For this review, take the finished solid that the model builds, in its own axes (mm). Face numbers are marked on the shaded views. A direction names the side the tool comes from. Round coordinates to 2 decimals unless told otherwise and drop trailing zeros. Loops run counter-clockwise (first coordinate to the right, second up) from the corner with the lowest first, then second, coordinate; pieces in that order, holes last. Notation, with made-up numbers: M 23.5,61 L 44.5,61 A12 ccw 44.5,82 Z; hole C 8.25,-26 d4. An arc over 180 degrees is marked long. Write item = value, one per line. Start each with the question number.
Autodesk Inventor part; units mm, degrees
ref_plane "YZ Plane" through (0, 0, 0) normal (1, 0, 0) x (0, 1, 0)
ref_plane "XZ Plane" through (0, 0, 0) normal (0, 1, 0) x (-1, 0, 0)
ref_plane "XY Plane" through (0, 0, 0) normal (0, 0, 1) x (1, 0, 0)
sketch "Sketch1" plane through (0, 0, 0) normal (0, 0, 1) x (1, 0, 0)
  line L0 (-11.1369, 11.1369) -> (11.1369, 11.1369) construction
  line L1 (11.1369, 11.1369) -> (11.1369, -11.1369) construction
  line L2 (11.1369, -11.1369) -> (-11.1369, -11.1369) construction
  line L3 (-11.1369, -11.1369) -> (-11.1369, 11.1369) construction
  line L4 (-11.1369, 11.1369) -> (11.1369, -11.1369) construction
  line L5 (11.1369, 11.1369) -> (-11.1369, -11.1369) construction
  circle A0 centre (-11.1369, 11.1369) radius 3
  circle A1 centre (11.1369, 11.1369) radius 3
  circle A2 centre (-11.1369, -11.1369) radius 3
  circle A3 centre (0, -15.6056) radius 3
  circle A4 centre (11.1369, -11.1369) radius 3
  line L6 (-11.1369, -11.1369) -> (0, -15.6056) construction
  line L7 (0, -15.6056) -> (11.1369, -11.1369) construction
  line L8 (0, 0) -> (0, 30.7503) construction
  circle A5 centre (-11.1369, 11.1369) radius 6
  circle A6 centre (-11.1369, -11.1369) radius 6
  circle A7 centre (11.1369, -11.1369) radius 6
  circle A8 centre (11.1369, 11.1369) radius 6
  line L9 (-19.2384, -29.2384) -> (19.2384, -29.2384)
  line L10 (29.2384, -19.2384) -> (29.2384, 19.2384)
  line L11 (19.2384, 29.2384) -> (-19.2384, 29.2384)
  line L12 (-29.2384, 19.2384) -> (-29.2384, -19.2384)
  line L13 (-29.2384, -29.2384) -> (29.2384, 29.2384) construction
  line L14 (29.2384, -29.2384) -> (-29.2384, 29.2384) construction
  line L15 (-29.2384, 19.2384) -> (-19.2384, 29.2384)
  line L16 (19.2384, 29.2384) -> (29.2384, 19.2384)
  line L17 (29.2384, -19.2384) -> (19.2384, -29.2384)
  line L18 (-19.2384, -29.2384) -> (-29.2384, -19.2384)
  circle A9 centre (0, 0) radius 35 construction
  point P0 (0, 0)
  point P1 (25, 0)
  point P2 (0, 0)
  dimension "d31" = 70
  dimension "d2" = 31.5
  dimension "d4" = 6
  dimension "d5" = 6
  dimension "d6" = 12
  dimension "d18" = 12
  dimension "d21" = 10
  dimension "d22" = 10
  dimension "d23" = 10
  dimension "d24" = 10
  dimension "d25" = 10
  dimension "d26" = 10
  dimension "d27" = 10
  dimension "d28" = 10
extrude "Extrusion1" add sketch "Sketch1" against normal blind 10 contours A5 | A6 | A7 | A8 | L18 L12 L15 L11 L16 L10 L17 L9
extrude "Extrusion3" cut sketch "Sketch1" against normal blind 5 contours A0 | A1 | A2 | A4 | A5 | A6 | A7 | A8
sketch "Sketch3" plane through (0, 0, 0) normal (0, 0, 1) x (1, 0, 0)
  circle A0 centre (-11.1369, -11.1369) radius 6
  circle A1 centre (11.1369, -11.1369) radius 6
  circle A2 centre (-11.1369, 11.1369) radius 6
  circle A3 centre (11.1369, 11.1369) radius 6
  line L0 (-29.2384, -19.2384) -> (-19.2384, -29.2384)
  line L1 (-19.2384, -29.2384) -> (19.2384, -29.2384)
  line L2 (19.2384, -29.2384) -> (29.2384, -19.2384)
  line L3 (29.2384, -19.2384) -> (29.2384, 19.2384)
  line L4 (29.2384, 19.2384) -> (19.2384, 29.2384)
  line L5 (19.2384, 29.2384) -> (-19.2384, 29.2384)
  line L6 (-19.2384, 29.2384) -> (-29.2384, 19.2384)
  line L7 (-29.2384, 19.2384) -> (-29.2384, -19.2384)
  circle A4 centre (0, -15.6056) radius 3
  line L8 (19.2384, 29.2384) -> (16.41, 26.41)
  line L9 (13.5815, 23.5815) -> (23.5815, 13.5815)
  line L10 (23.5815, 13.5815) -> (26.41, 16.41) construction
  line L11 (29.2384, 19.2384) -> (29.2384, -19.2384)
  line L12 (29.2384, 19.2384) -> (19.2384, 29.2384)
  line L13 (23.5815, 13.5815) -> (23.5815, 5.1369)
  circle A5 centre (11.1369, 11.1369) radius 6
  line L14 (26.41, 16.41) -> (26.41, 2.5685)
  line L15 (26.41, 16.41) -> (29.2384, 19.2384)
  line L16 (17.1369, 11.1369) -> (17.1369, 5.1369)
  line L17 (17.1369, 5.1369) -> (23.5815, 5.1369)
  line L18 (0, 0) -> (17.1369, 0) construction
  line L19 (16.41, 26.41) -> (2.5685, 26.41)
  line L20 (0, 17.1369) -> (0, 0) construction
  line L21 (16.41, 26.41) -> (13.5815, 23.5815) construction
  line L22 (13.5815, 23.5815) -> (5.1369, 23.5815)
  line L23 (5.1369, 23.5815) -> (5.1369, 17.1369)
  line L24 (5.1369, 17.1369) -> (11.1369, 17.1369)
  circle A6 centre (11.1369, 11.1369) radius 6
  line L25 (0, 17.1369) -> (0, 29.2384)
  line L26 (19.2384, 29.2384) -> (-19.2384, 29.2384)
  line L27 (17.1369, 0) -> (29.2384, 0)
  line L28 (2.5685, 17.1369) -> (2.5685, 26.41)
  line L29 (0, 17.1369) -> (2.5685, 17.1369)
  line L30 (2.5685, 17.1369) -> (5.1369, 17.1369) construction
  line L31 (26.41, 2.5685) -> (17.1369, 2.5685)
  line L32 (17.1369, 2.5685) -> (17.1369, 0)
  line L33 (17.1369, 2.5685) -> (17.1369, 5.1369) construction
  dimension "d38" = 8
extrude "Extrusion5" cut sketch "Sketch3" against normal through all contours A3 L24 L23 L22 L9 L13 L17 L16 | L5 L8 L19 L28 L29 L25 | L27 L32 L31 L14 L15 L3
sketch "Sketch4" plane through (0, 0, -5) normal (0, 0, 1) x (1, 0, 0)
  circle A0 centre (11.1369, 11.1369) radius 3
  arc A1 (11.1369, 17.1369) -> (17.1369, 11.1369) centre (11.1369, 11.1369) ccw
  arc A2 (17.1369, 11.1369) -> (11.1369, 17.1369) centre (11.1369, 11.1369) ccw
  line L0 (17.1369, 11.1369) -> (17.1369, 5.1369)
  line L1 (17.1369, 5.1369) -> (17.1369, 11.1369)
  line L2 (5.1369, 17.1369) -> (11.1369, 17.1369)
  line L3 (11.1369, 17.1369) -> (5.1369, 17.1369)
  line L4 (17.1369, 5.1369) -> (11.1369, 5.1369)
  line L5 (5.1369, 17.1369) -> (11.1369, 17.1369)
  line L6 (5.1369, 17.1369) -> (5.1369, 11.1369)
  point P0 (0, 0)
extrude "Extrusion6" cut sketch "Sketch4" along normal through all contours A1 L6 L2 | L0 L4 A1
pattern_circular "Circular Pattern2" count 4 over 360 about axis through (0, 0, -10) along (0, 0, 1) of "Extrusion5", "Extrusion6"
sketch "Sketch2" plane through (29.2384, 19.2384, -10) normal (0.7071, 0.7071, 0) x (-0.7071, 0.7071, 0)
  line L0 (0, 10) -> (0, 0) construction
  line L1 (14.1421, 0) -> (0, 0) construction
  line L2 (14.1421, 10) -> (14.1421, 0) construction
  line L3 (0, 10) -> (14.1421, 10) construction
  line L4 (14.1421, 10) -> (0, 0) construction
  circle A0 centre (7.0711, 5) radius 2
  point P0 (7.0711, 10)
  dimension "d32" = 4
extrude "Extrusion4" cut sketch "Sketch2" against normal up to next
pattern_circular "Circular Pattern1" count 4 over 360 about axis through (0, 0, -10) along (0, 0, 1) of "Extrusion4"
equation "\"d22\" = d21"
equation "\"d23\" = d21"
equation "\"d24\" = d23"
equation "\"d25\" = d21"
equation "\"d26\" = d25"
equation "\"d27\" = d21"
equation "\"d28\" = d27"
properties part number "Interface Block" material "ABS Plastic"
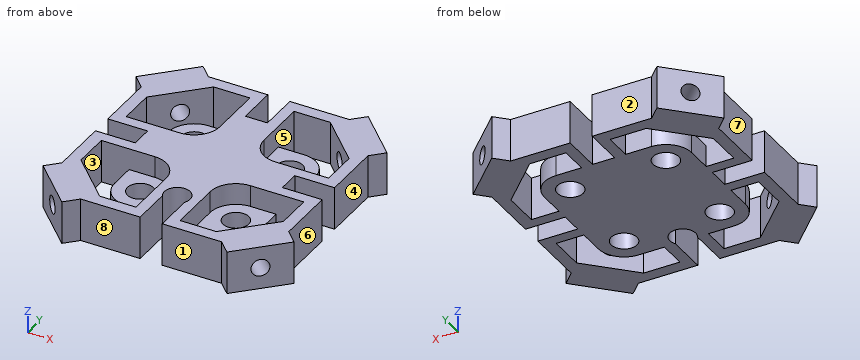
(1) Draft analysis for pull direction X (two halves, no side actions). For the marked faces 6, 7 and 8, state which applies: +X half, -X half, draft (parallel to the pull), parting line (faces both ways), or undercut.
(2) Add section B-B on z = -2. Count the separate pieces of the cut face and the enclosed holes in it, and give its area (3 significant figures).
(3) Tool access review of the marked faces 1, 2, 3, 4 and 5: name each direction out of +Z, -Z, +X, -X, +Y, -Y from which nothing blocks a thin tool from reaching the whole face with its end or side.
(4) Add section D-D on x = 0. Write out the cut boundary in (y, z), and give its area (3 significant figures).
(5) Add section C-C on y = 3.5. Write out the cut boundary in (x, z), and give its area (3 significant figures).
(6) Add section A-A on x = -7. Write out the cut boundary in (y, z).
(7) For pin 1 Ø3 at (y, z) = (-17, -3) entering from +X; pin 2 Ø2.5 at (y, z) = (-7, -6.5) entering from -X; pin 3 Ø4 at (y, z) = (-8.5, -6.5) entering from +X; pin 4 Ø5 at (x, y) = (11.14, 11.14) entering from +Z, all flat-tipped, find the tip position at first contact; note any pin that passes through.
(8) Wall thickness on L1, parallel to X at y = 6.5, z = -8.75; L2, parallel to Y at x = -11, z = -9: over which ranges is each line inside the solid? List them lowest first.
Answer sheet:
q1.face_6 = +X half
q1.face_7 = -X half
q1.face_8 = undercut
q2.separate_pieces = 1
q2.enclosed_holes = 4
q2.area = 1,470 mm²
q3.face_1 = +Z, -Z, -Y
q3.face_2 = +Z, -Z, +Y
q3.face_3 = +Z, -Z
q3.face_4 = +Z, -Z, +X
q3.face_5 = +Z
q4.outline = M -12.61,-10 L 17.14,-10 L 17.14,0 L -12.61,0 Z
q4.area = 297 mm²
q5.outline = M -26.41,-10 L 26.41,-10 L 26.41,0 L -26.41,0 Z
q5.area = 528 mm²
q6.outline = M -26.41,-10 L -23.58,-10 L -23.58,0 L -26.41,0 Z; M -17.14,-10 L 17.14,-10 L 17.14,-5 L 6.79,-5 L 6.79,0 L -6.79,0 L -6.79,-5 L -17.14,-5 Z; M 23.58,-10 L 26.41,-10 L 26.41,0 L 23.58,0 Z
q7.pin_1 = 28.5
q7.pin_2 = -26.41
q7.pin_3 = 26.41
q7.pin_4 = through
q8.L1 = -26.41 to -23.58, -17.14 to 17.14, 23.58 to 26.41
q8.L2 = -26.41 to -23.58, -17.14 to -14.13, -8.14 to 8.14, 14.13 to 17.14, 23.58 to 26.41
